from build123d import *

# Parameters (mm, degrees)
BOSS_EXTRU_1_CORPS_DEPTH    = 335
CONG_1_R                    = 1.5
CONG_2_R                    = 0.4
CONG_4_R                    = 1
CONG_1_OF_SYM_TRIE_BRAS_R   = 1.5
CONG_2_OF_SYM_TRIE_BRAS_R   = 0.4
CONG_4_OF_SYM_TRIE_BRAS_R   = 1
SYM_TRIE_BRAS_DOUBLE_DEPTH  = 335
APR_S_TARODAGE_M6_R         = 3
ENL_V_MAT_FILETAGE_M6_DEPTH = 336.298374586


# Read off the part's stored shape, not the designer's step: Symétrie Bras double
with BuildPart() as part:
    # Esquisse4 → Boss.-Extru.1 Corps (new body)
    with BuildSketch(Plane(origin=(0, 0, 0), x_dir=(1, 0, 0), z_dir=(0, 1, 0))):
        Polygon((0, 0), (-4.5, 0), (-4.5, 3.625), (-6.875, 6), (-8.5, 6), (-8.5, 3), (-9.5, 3), (-9.5, 3.5), (-10, 3.5), (-10, 10), (-3.5, 10), (-3.5, 9.5), (-3, 9.5), (-3, 8.5), (-6, 8.5), (-6, 6.875), (-3.625, 4.5), (0, 4.5), align=None)
    boss_extru_1_corps = extrude(amount=BOSS_EXTRU_1_CORPS_DEPTH)

    # Congé1
    cong_1_edges = [part.edges().sort_by_distance(p)[0] for p in [
        (-10, 167.5, -10),
    ]]
    fillet(cong_1_edges, radius=CONG_1_R)

    # Congé2
    cong_2_edges = [part.edges().sort_by_distance(p)[0] for p in [
        (-8.5, 167.5, -6),
        (-6, 167.5, -8.5),
    ]]
    fillet(cong_2_edges, radius=CONG_2_R)

    # Congé4
    cong_4_edges = [part.edges().sort_by_distance(p)[0] for p in [
        (-4.5, 167.5, -3.625),
        (-6.875, 167.5, -6),
        (-6, 167.5, -6.875),
        (-3.625, 167.5, -4.5),
    ]]
    fillet(cong_4_edges, radius=CONG_4_R)

    # Symétrie Bras: Boss.-Extru.1 Corps across plane
    add(boss_extru_1_corps.mirror(Plane(origin=(0, 335, -4.5), x_dir=(0, 0, 1), z_dir=(-1, 0, 0))))

    # Congé1 of Symétrie Bras
    cong_1_of_sym_trie_bras_edges = [part.edges().sort_by_distance(p)[0] for p in [
        (10, 167.5, -10),
    ]]
    fillet(cong_1_of_sym_trie_bras_edges, radius=CONG_1_OF_SYM_TRIE_BRAS_R)

    # Congé2 of Symétrie Bras
    cong_2_of_sym_trie_bras_edges = [part.edges().sort_by_distance(p)[0] for p in [
        (8.5, 167.5, -6),
        (6, 167.5, -8.5),
    ]]
    fillet(cong_2_of_sym_trie_bras_edges, radius=CONG_2_OF_SYM_TRIE_BRAS_R)

    # Congé4 of Symétrie Bras
    cong_4_of_sym_trie_bras_edges = [part.edges().sort_by_distance(p)[0] for p in [
        (4.5, 167.5, -3.625),
        (6.875, 167.5, -6),
        (6, 167.5, -6.875),
        (3.625, 167.5, -4.5),
    ]]
    fillet(cong_4_of_sym_trie_bras_edges, radius=CONG_4_OF_SYM_TRIE_BRAS_R)

    # Symétrie Bras double outline → Symétrie Bras double (add)
    with BuildSketch(Plane(origin=(0, 0, 0), x_dir=(1, 0, 0), z_dir=(0, 1, 0))):
        with BuildLine():
            ThreePointArc((7.289213562, -6), (6.90653013, -5.923879533), (6.582106781, -5.707106781))
            Line((6.582106781, -5.707106781), (4.792893219, -3.917893219))
            ThreePointArc((4.792893219, -3.917893219), (4.576120467, -3.59346987), (4.5, -3.210786438))
            Line((4.5, -3.210786438), (4.5, 0))
            Line((4.5, 0), (-4.5, 0))
            Line((-4.5, 0), (-4.5, -3.210786438))
            ThreePointArc((-4.5, -3.210786438), (-4.576120467, -3.59346987), (-4.792893219, -3.917893219))
            Line((-4.792893219, -3.917893219), (-6.582106781, -5.707106781))
            ThreePointArc((-6.582106781, -5.707106781), (-6.90653013, -5.923879533), (-7.289213562, -6))
            Line((-7.289213562, -6), (-8.1, -6))
            ThreePointArc((-8.1, -6), (-8.382842712, -5.882842712), (-8.5, -5.6))
            Line((-8.5, -5.6), (-8.5, -3))
            Line((-8.5, -3), (-9.5, -3))
            Line((-9.5, -3), (-9.5, -3.5))
            Line((-9.5, -3.5), (-10, -3.5))
            Line((-10, -3.5), (-10, -8.5))
            ThreePointArc((-10, -8.5), (-9.560660172, -9.560660172), (-8.5, -10))
            Line((-8.5, -10), (-3.5, -10))
            Line((-3.5, -10), (-3.5, -9.5))
            Line((-3.5, -9.5), (-3, -9.5))
            Line((-3, -9.5), (-3, -8.5))
            Line((-3, -8.5), (-5.6, -8.5))
            ThreePointArc((-5.6, -8.5), (-5.882842712, -8.382842712), (-6, -8.1))
            Line((-6, -8.1), (-6, -7.289213562))
            ThreePointArc((-6, -7.289213562), (-5.923879533, -6.90653013), (-5.707106781, -6.582106781))
            Line((-5.707106781, -6.582106781), (-3.917893219, -4.792893219))
            ThreePointArc((-3.917893219, -4.792893219), (-3.59346987, -4.576120467), (-3.210786438, -4.5))
            Line((-3.210786438, -4.5), (3.210786438, -4.5))
            ThreePointArc((3.210786438, -4.5), (3.59346987, -4.576120467), (3.917893219, -4.792893219))
            Line((3.917893219, -4.792893219), (5.707106781, -6.582106781))
            ThreePointArc((5.707106781, -6.582106781), (5.923879533, -6.90653013), (6, -7.289213562))
            Line((6, -7.289213562), (6, -8.1))
            ThreePointArc((6, -8.1), (5.882842712, -8.382842712), (5.6, -8.5))
            Line((5.6, -8.5), (3, -8.5))
            Line((3, -8.5), (3, -9.5))
            Line((3, -9.5), (3.5, -9.5))
            Line((3.5, -9.5), (3.5, -10))
            Line((3.5, -10), (8.5, -10))
            ThreePointArc((8.5, -10), (9.560660172, -9.560660172), (10, -8.5))
            Line((10, -8.5), (10, -3.5))
            Line((10, -3.5), (9.5, -3.5))
            Line((9.5, -3.5), (9.5, -3))
            Line((9.5, -3), (8.5, -3))
            Line((8.5, -3), (8.5, -5.6))
            ThreePointArc((8.5, -5.6), (8.382842712, -5.882842712), (8.1, -6))
            Line((8.1, -6), (7.289213562, -6))
        make_face()
    extrude(amount=SYM_TRIE_BRAS_DOUBLE_DEPTH)

    # Après tarodage M6 → Enlèv. mat.-Filetage M6 (cut, through all)
    with BuildSketch(Plane.XZ):
        with Locations(Location((0, 0, 0), (0, 0, 270))):
            Circle(APR_S_TARODAGE_M6_R)
    extrude(amount=-ENL_V_MAT_FILETAGE_M6_DEPTH, mode=Mode.SUBTRACT)


solid = part.part
Can you work these out from the model? Positions are in its coordinate system, mm. Coordinates: 2 decimals unless noted, no trailing zeros. Loops run counter-clockwise (first coordinate to the right, second up) from the corner with the lowest first, then second, coordinate; pieces in that order, holes last. Notation, with made-up numbers: (66.5, 17.5) - (100.5, 17.5) arc R13 cw to (100.5, 23.5) - close; hole circle Ø3 at (-25.5, 54). An arc over 180 degrees is marked (long way). Answer as a JSON object with one key per item and string values. Group by question number.
Item 1: For pin 1 (1.9 mm diameter, centred on y = 164.5, z = 1, fed in from +X); pin 2 (0.8 mm diameter, centred on x = 9, y = 117.5, fed in from -Z); pin 3 (0.6 mm diameter, centred on y = 248, z = -10, fed in from -X), each with a flat end and sliding along its axis, tell me the tip position at first contact or that it passes through.
Item 2: If we mould it in two halves opening along X, with no side actions, what happens to faces 1 (the face through (0, 165, 4.5)), 2 (the face through (2.1, 0, -2.4))? For each: released by +X, released by -X, zero draft, split by the parting line, or undercut.
Item 3: If we section it at A-A (z = 0): List the corners of the cut face in (x, y) for me, plus the area to 4 significant figures.
Item 4: If we section it at B-B (x = 0): List the corners of the cut face in (y, z) for me, plus the area to 4 significant figures.
Item 5: If I drill on L1, parallel to X at y = 91, z = 0; L2, parallel to Z at x = 6.5, y = 78 (3 decimals); L3, parallel to X at y = 244, z = 7.5, over which ranges is the centre line in solid material (lowest first)? Write a range as from..to.
Returned:
{
 "1": {"pin 1": "stops at x = 4.5", "pin 2": "stops at z = -10", "pin 3": "stops at x = -9.4"},
 "2": {"face 1": "undercut", "face 2": "zero draft"},
 "3": {"outline": "(-4.5, 0) - (-3, 0) - (-3, 335) - (-4.5, 335) - close; (3, 0) - (4.5, 0) - (4.5, 335) - (3, 335) - close", "area": "1,005 mm²"},
 "4": {"outline": "(0, -4.5) - (335, -4.5) - (335, -3) - (0, -3) - close; (0, 3) - (335, 3) - (335, 4.5) - (0, 4.5) - close", "area": "1,005 mm²"},
 "5": {"L1": "x = -4.5..-3, 3..4.5", "L2": "z = -10..-5.625, 5.625..10", "L3": "x = -10..-6, 6..10"}
}
